Read the model definition and answer for the solid it produces. Units are mm, in the model's axes. Face numbers are marked on the shaded views. A direction names the side the tool comes from. Give positions to 0.01 mm unless a question says otherwise; leave off trailing zeros. Order: outer loops, then holes, each group sorted by start corner. A loop starts at its lowest first (then second) coordinate and runs counter-clockwise, first axis right, second up. Notation, with made-up numbers: (82, 51.25) -> (103, 51.25) arc R28 cw to (103, 71.25) -> close; hole circle Ø5 at (70.25, 72). An arc over 180 degrees is marked (long way). Answer as CSV lines item,"result". Start each with the question number.
1) Find section A-A (y = -8.5). Determine the outline of the cut face in (x, z), and give its area (3 significant figures).
2) Flat-ended cylindrical pins translate along their axes: pin 1 Ø2.5 at (x, z) = (-292.5, 1.5) entering from -Y; pin 2 Ø5 at (y, z) = (-10.5, -2) entering from +X. Find the tip coordinate at first contact, or state that the pin passes through.
3) Find section B-B (x = -145). Determine the outline of the cut face in (y, z).
4) Straight lines are drawn through the part: L1, parallel to X at y = 4.75, z = 0; L2, parallel to X at y = -8.25, z = -2.5; L3, parallel to X at y = 1.5, z = 2.5. For each, find the intervals that lie inside material, in ascending order. Write a range as from..to.
5) The mould has two halves that part along X. Classify the marked faces 1, 2 and 3: +X half, -X half, draft (parallel to the pull), parting line (faces both ways), or undercut.
6) Find section D-D (x = -229.5). Determine the outline of the cut face in (y, z).
7) Find section C-C (z = 0). State how many separate pieces and enclosed holes the cut face has, and give its area (3 significant figures).
8) For the marked faces 4, 5 and 6, determine the directions among +Z, -Z, +X, -X, +Y, -Y from which every point of the face is accessible in a straight line to the end or side of a thin tool.
```python
from build123d import *

# Parameters (mm, degrees)
SKETCH1_W           = 170
SKETCH1_H           = 10
BOSS_EXTRUDE1_DEPTH = 6
SKETCH3_W           = 3
SKETCH3_H           = 10
BOSS_EXTRUDE2_DEPTH = 15
LPATTERN1_COUNT     = 6
LPATTERN1_PITCH     = 28.3
SKETCH5_R           = 3
SKETCH5_R_2         = 1.8
CUT_EXTRUDE1_DEPTH  = 10
SKETCH7_W           = 15.610569604
SKETCH7_H           = 29.423295864
SKETCH7_W_2         = 14.543842925
SKETCH7_H_2         = 20.261696827
SKETCH7_W_3         = 15.463066773
SKETCH7_H_3         = 26.876388592
CUT_EXTRUDE3_DEPTH  = 3


with BuildPart() as part:
    # Sketch1 → Boss-Extrude1 (new body)
    with BuildSketch(Plane(origin=(0, 0, 0), x_dir=(1, 0, 0), z_dir=(0, 1, 0))):
        with Locations((-215, 0)):
            Rectangle(SKETCH1_W, SKETCH1_H)
    extrude(amount=BOSS_EXTRUDE1_DEPTH)

    # Sketch3 → Boss-Extrude2 (add)
    with BuildSketch(Plane.XZ):
        with Locations((-298.5, 0)):
            Rectangle(SKETCH3_W, SKETCH3_H)
    boss_extrude2 = extrude(amount=BOSS_EXTRUDE2_DEPTH)

    # LPattern1: Boss-Extrude2 ×6
    with Locations(*[(i * LPATTERN1_PITCH, 0, 0) for i in range(1, LPATTERN1_COUNT)]):
        add(boss_extrude2)

    # Sketch5 → Cut-Extrude1 (cut)
    with BuildSketch(Plane(origin=(0, 6, 0), x_dir=(1, 0, 0), z_dir=(0, 1, 0))):
        with Locations((-225, 0)):
            Circle(SKETCH5_R)
        with Locations((225, 0)):
            Circle(SKETCH5_R_2)
        with Locations((165, 0)):
            Circle(SKETCH5_R_2)
        with Locations((-280, 0)):
            Circle(SKETCH5_R)
        with Locations((-145, 0)):
            Circle(SKETCH5_R)
    extrude(amount=-CUT_EXTRUDE1_DEPTH, mode=Mode.SUBTRACT)

    # Sketch7 → Cut-Extrude3 (cut)
    with BuildSketch(Plane.XZ):
        with Locations((-280.60295859, 0.084727736)):
            Rectangle(SKETCH7_W, SKETCH7_H)
        with Locations((-225.915608204, -0.229636086)):
            Rectangle(SKETCH7_W_2, SKETCH7_H_2)
        with Locations((-144.85630026, -0.160459025)):
            Rectangle(SKETCH7_W_3, SKETCH7_H_3)
    extrude(amount=-CUT_EXTRUDE3_DEPTH, mode=Mode.SUBTRACT)


solid = part.part
```
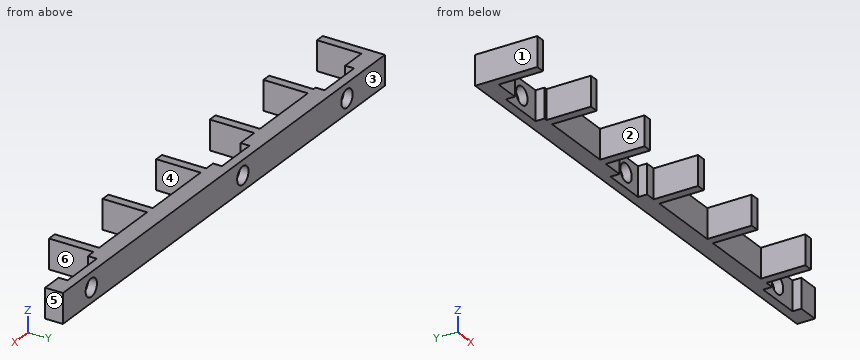
Findings below:
1,outline,"(-300, -5) -> (-297, -5) -> (-297, 5) -> (-300, 5) -> close; (-271.7, -5) -> (-268.7, -5) -> (-268.7, 5) -> (-271.7, 5) -> close; (-243.4, -5) -> (-240.4, -5) -> (-240.4, 5) -> (-243.4, 5) -> close; (-215.1, -5) -> (-212.1, -5) -> (-212.1, 5) -> (-215.1, 5) -> close; (-186.8, -5) -> (-183.8, -5) -> (-183.8, 5) -> (-186.8, 5) -> close; (-158.5, -5) -> (-155.5, -5) -> (-155.5, 5) -> (-158.5, 5) -> close"
1,area,"180 mm²"
2,pin 1,"y = 0"
2,pin 2,"x = -155.5"
3,outline,"(3, -5) -> (6, -5) -> (6, -3) -> (3, -3) -> close; (3, 3) -> (6, 3) -> (6, 5) -> (3, 5) -> close"
4,L1,"-300..-283, -277..-228, -222..-148, -142..-130"
4,L2,"-300..-297, -271.7..-268.7, -243.4..-240.4, -215.1..-212.1, -186.8..-183.8, -158.5..-155.5"
4,L3,"-300..-288.41, -272.8..-233.19, -218.64..-152.59, -137.12..-130"
5,face 1,"-X half"
5,face 2,"undercut"
5,face 3,"draft"
6,outline,"(3, -5) -> (6, -5) -> (6, 5) -> (3, 5) -> close"
7,separate pieces,"4"
7,enclosed holes,"0"
7,area,"1,100 mm²"
8,face 4,"+Z, -Z, -Y"
8,face 5,"+Z, -Z, +X, +Y, -Y"
8,face 6,"+Z, -Z, +X, -Y"
